```python
from build123d import *

# Parameters (mm, degrees)
CROQUIS1_W              = 35
CROQUIS1_H              = 20
SALIENTE_EXTRUIR1_DEPTH = 7
REDONDEO1_R             = 2


with BuildPart() as part:
    # Croquis1 → Saliente-Extruir1 (new body)
    with BuildSketch(Plane(origin=(0, 0, 0), x_dir=(1, 0, 0), z_dir=(0, 1, 0))):
        Rectangle(CROQUIS1_W, CROQUIS1_H)
    extrude(amount=SALIENTE_EXTRUIR1_DEPTH)

    # Redondeo1
    redondeo1_edges = [part.edges().sort_by_distance(p)[0] for p in [
        (-17.5, 7, 0),
        (0, 7, 10),
        (17.5, 7, 0),
        (0, 0, 10),
        (0, 0, -10),
        (17.5, 0, 0),
        (0, 7, -10),
        (17.5, 3.5, 10),
        (-17.5, 3.5, 10),
        (-17.5, 3.5, -10),
        (17.5, 3.5, -10),
    ]]
    fillet(redondeo1_edges, radius=REDONDEO1_R)


solid = part.part
```
Work out the finished part from the listing and answer in its coordinate system (mm). Give positions to 0.01 mm unless a question says otherwise; leave off trailing zeros. Order: outer loops, then holes, each group sorted by start corner. A loop starts at its lowest first (then second) coordinate and runs counter-clockwise, first axis right, second up. Notation, with made-up numbers: M 40.5,30.5 L 82.5,30.5 A22 ccw 82.5,57.5 Z; hole C 78.5,-10 d6. An arc over 180 degrees is marked long. Return JSON: item names as keys, results as strings.
1) Section A-A, the plane x = 7 is taken. Write down the section's boundary in (y, z), plus the area to 3 significant figures.
Resolved:
{"outline": "M 0,-8 A2 ccw 2,-10 L 5,-10 A2 ccw 7,-8 L 7,8 A2 ccw 5,10 L 2,10 A2 ccw 0,8 Z", "area": "137 mm^2"}
2) Section B-B, the plane y = 1.25 is taken. Write down the section's boundary in (x, z), plus the area to 3 significant figures.
Resolved:
{"outline": "M -17.5,-8 A2 ccw -16.25,-9.85 L 15.5,-9.85 A1.85 ccw 17.35,-8 L 17.35,8 A1.85 ccw 15.5,9.85 L -16.25,9.85 A2 ccw -17.5,8 Z", "area": "684 mm^2"}
3) Straight lines are drawn through the part: line 1 along Z through (x, y) = (-13, 6); line 2 along Z through (x, y) = (10, 5.5); line 3 along X through (y, z) = (5.75, 0.5). For each, find the intervals that lie inside material, in ascending order. Write a range as [from, to].
Resolved:
{"line 1": "[-9.73, 9.73]", "line 2": "[-9.94, 9.94]", "line 3": "[-17.35, 17.35]"}
